Print and shaded views of the part. All mm, measured from the part's lowest x, y and z. Give positions to 0.01 mm unless a question says otherwise; leave off trailing zeros. Order: outer loops, then holes, each group sorted by start corner. A loop starts at its lowest first (then second) coordinate and runs counter-clockwise, first axis right, second up. Notation, with made-up numbers: (74, 68.5) - (97, 68.5) arc R13 cw to (97, 81.5) - close; hole circle Ø3 at (11.5, 36.25). An arc over 180 degrees is marked (long way). Answer in a Markdown table with one row per item.
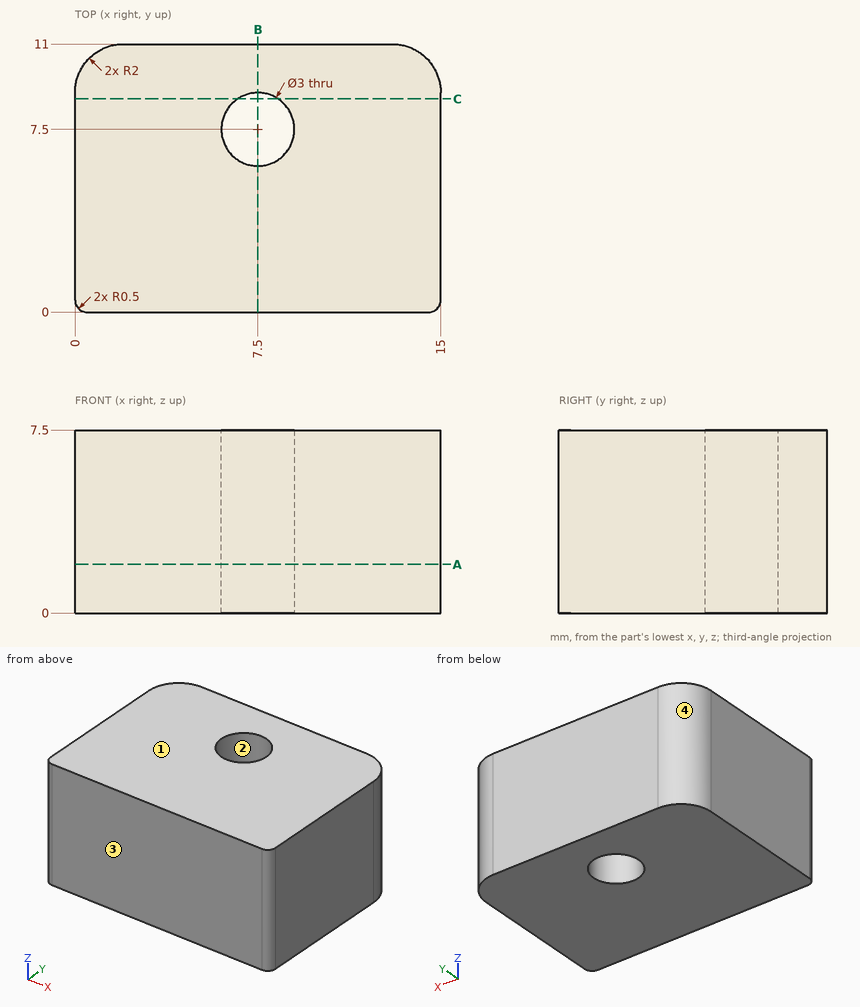
1. Cut at B-B on x = 7.5. Write the cut outline in (y, z), and give its area (3 significant figures).
Check result:
| item | result |
|---|---|
| outline | (0, 0) - (6, 0) - (6, 7.5) - (0, 7.5) - close; (9, 0) - (11, 0) - (11, 7.5) - (9, 7.5) - close |
| area | 60.0 mm² |
2. Cut at A-A on z = 2. Write the cut outline in (x, y).
Check result:
| item | result |
|---|---|
| outline | (0, 0.5) arc R0.5 ccw to (0.5, 0) - (14.5, 0) arc R0.5 ccw to (15, 0.5) - (15, 9) arc R2 ccw to (13, 11) - (2, 11) arc R2 ccw to (0, 9) - close; hole circle Ø3 at (7.5, 7.5) |
3. Probe line 1 (Y direction, x = 7.5, z = 2); line 2 (X direction, y = 7.25, z = 5); line 3 (Y direction, x = 8.5, z = 1.75). List the from-to ranges inside material, lowest first.
Check result:
| item | result |
|---|---|
| line 1 | y = 0 to 6, 9 to 11 |
| line 2 | x = 0 to 6.02, 8.98 to 15 |
| line 3 | y = 0 to 6.38, 8.62 to 11 |
4. Two-plate mould, pull along Y, no slides. Class the marked faces 1, 2, 3 and 4: +Y half, -Y half, draft (parallel to the pull), parting line (faces both ways), or undercut.
Check result:
| item | result |
|---|---|
| face 1 | draft |
| face 2 | undercut |
| face 3 | -Y half |
| face 4 | +Y half |
5. Cut at C-C on y = 8.75. Write the cut outline in (x, z), and give its area (3 significant figures).
Check result:
| item | result |
|---|---|
| outline | (0, 0) - (6.67, 0) - (6.67, 7.5) - (0, 7.5) - close; (8.33, 0) - (15, 0) - (15, 7.5) - (8.33, 7.5) - close |
| area | 100 mm² |
